Here's how the part is built. I have some questions about the finished solid (model axes, mm). A direction names the side the tool comes from. Round coordinates to 2 decimals unless told otherwise and drop trailing zeros. Loops run counter-clockwise (first coordinate to the right, second up) from the corner with the lowest first, then second, coordinate; pieces in that order, holes last. Notation, with made-up numbers: M -25,-7 L -17,-7 A21 ccw -17,17 Z; hole C 3,61 d11. An arc over 180 degrees is marked long. Answer as CSV lines item,"result".
```python
from build123d import *

# Parameters (mm, degrees)
SKETCH_2_W          = 14.6
SKETCH_2_H          = 56.56
SKETCH_2_R          = 0.25
SKETCH_2_W_2        = 8.75
SKETCH_2_H_2        = 1
EXTRUDE_1_DEPTH     = 1.6
SKETCH_3_W          = 2.7
SKETCH_3_H          = 11.6
CUT_EXTRUDE_1_DEPTH = 1.6
FILLET_2_R          = 1


with BuildPart() as part:
    # 草图2 → 凸台-拉伸1 (new body)
    with BuildSketch(Plane.XY):
        with Locations((-0.85, 5.8)):
            Rectangle(SKETCH_2_W, SKETCH_2_H)
        with Locations((0.35, 28.78)):
            Circle(SKETCH_2_R, mode=Mode.SUBTRACT)
        with Locations((0.25, -9.98)):
            Rectangle(SKETCH_2_W_2, SKETCH_2_H_2, mode=Mode.SUBTRACT)
    extrude(amount=EXTRUDE_1_DEPTH)

    # 草图3 → 切除-拉伸1 (cut)
    with BuildSketch(Plane(origin=(0, 0, 0), x_dir=(-1, 0, 0), z_dir=(0, 0, -1))):
        with Locations((6.8, 28.28)):
            Rectangle(SKETCH_3_W, SKETCH_3_H)
    extrude(amount=-CUT_EXTRUDE_1_DEPTH, mode=Mode.SUBTRACT)

    # 圆角2
    fillet_2_edges = [part.edges().sort_by_distance(p)[0] for p in [
        (-5.45, 22.48, 0.8),
        (-5.45, 34.08, 0.8),
        (-8.15, 22.48, 0.8),
        (6.45, -22.48, 0.8),
        (-8.15, -22.48, 0.8),
        (6.45, 34.08, 0.8),
    ]]
    fillet(fillet_2_edges, radius=FILLET_2_R)


solid = part.part
```
1. I want a section at B-B, the plane z = 1.3. Please give me the cut outline in (x, y) (3 decimals), and give its area (3 significant figures).
Evaluation:
outline,"M -8.15,-21.48 A1 ccw -7.15,-22.48 L 5.45,-22.48 A1 ccw 6.45,-21.48 L 6.45,33.08 A1 ccw 5.45,34.08 L -4.45,34.08 A1 ccw -5.45,33.08 L -5.45,23.48 A1 cw -6.45,22.48 L -7.15,22.48 A1 ccw -8.15,21.48 Z; hole M -4.125,-10.48 L 4.625,-10.48 L 4.625,-9.48 L -4.125,-9.48 Z; hole C 0.35,28.78 d0.5"
area,"785 mm²"
2. I want a section at A-A, the plane x = 1.5. Please give me the cut outline in (y, z), and give its area (3 significant figures).
Evaluation:
outline,"M -22.48,0 L -10.48,0 L -10.48,1.6 L -22.48,1.6 Z; M -9.48,0 L 34.08,0 L 34.08,1.6 L -9.48,1.6 Z"
area,"88.9 mm²"
3. For P1, Ø5, axis at x = 0.5, y = 27.5, coming from the -Z side, with a flat end and sliding along its axis, tell me the tip position at first contact or that it passes through.
Evaluation:
P1,"stops at z = 0"
4. I want a section at C-C, the plane y = 28. Please give me the cut outline in (x, z), and give its area (3 significant figures).
Evaluation:
outline,"M -5.45,0 L 6.45,0 L 6.45,1.6 L -5.45,1.6 Z"
area,"19.0 mm²"
5. Which directions (+Z, -Z, +X, -X, +Y, -Y) give clear straight access to the entire face, cutting with the end or side of a thin tool? Please do faces 5 (the flat face through (0, -9.48, 1)), 6 (the flat face through (-8.15, 0, 1)).
Evaluation:
face 5,"+Z, -Z"
face 6,"+Z, -Z, -X, +Y, -Y"
6. If I drill on line 1 (Y direction, x = 0.35, z = 0.9); line 2 (Y direction, x = 4.5, z = 0.35); line 3 (X direction, y = 28.78, z = 0.9), over which ranges is the centre line in solid material (lowest first)? Write a range as [from, to].
Evaluation:
line 1,"y = [-22.48, -10.48], [-9.48, 28.53], [29.03, 34.08]"
line 2,"y = [-22.48, -10.48], [-9.48, 34.08]"
line 3,"x = [-5.45, 0.1], [0.6, 6.45]"
7. We'd pull the mould along X, two halves only. Please class faces 1 (the flat face through (-1, -22.48, 1)), 2 (the flat face through (-5.45, 28, 1)), 3 (the flat face through (0, -10.48, 1)), 4 (the flat face through (-4.125, -10, 1)): pulls with the +X half, pulls with the -X half, needs draft (parallel to the pull), parting line crosses it, or undercut.
Evaluation:
face 1,"needs draft"
face 2,"pulls with the -X half"
face 3,"undercut"
face 4,"undercut"
